from build123d import *

# Parameters (mm, degrees)
BOSS_EXTRUDE1_DEPTH     = 3.175
FILLET1_R               = 3.81
SKETCH2_R               = 2.032
CUT_EXTRUDE1_DEPTH      = 211.342252353
FILLET2_R               = 6.35
FILLET3_R               = 2.54
FILLET4_R               = 3.81
FILLET5_R               = 3.81
CUT_EXTRUDE2_DEPTH      = 211.342252353
CUT_EXTRUDE2_DEPTH_BACK = 211.342252353
FILLET6_R               = 5.08


with BuildPart() as part:
    # Sketch1 → Boss-Extrude1 (new body)
    with BuildSketch(Plane(origin=(0, 0, 0), x_dir=(1, 0, 0), z_dir=(0, 1, 0))):
        Polygon((50.8, 0), (0, 0), (0, -101.6), (50.8, -101.6), (50.8, -88.9), (63.5, -88.9), (63.5, -101.6), (120.65, -101.6), (120.65, -88.9), (133.35, -88.9), (133.35, -101.6), (184.15, -101.6), (184.15, 0), (133.35, 0), (133.35, -29.21), (120.65, -29.21), (120.65, -19.05), (63.5, -19.05), (63.5, -29.21), (50.8, -29.21), align=None)
    extrude(amount=BOSS_EXTRUDE1_DEPTH)

    # Fillet1
    fillet1_edges = [part.edges().sort_by_distance(p)[0] for p in [
        (0, 1.5875, 101.6),
        (0, 1.5875, 0),
        (184.15, 1.5875, 0),
        (184.15, 1.5875, 101.6),
    ]]
    fillet(fillet1_edges, radius=FILLET1_R)

    # Sketch2 → Cut-Extrude1 (cut, through all)
    with BuildSketch(Plane(origin=(0, 3.175, 0), x_dir=(1, 0, 0), z_dir=(0, 1, 0))):
        with Locations(Location((5.437401114, -89.146320086, 0), (0, 0, 270))):
            Circle(SKETCH2_R)
        with Locations(Location((178.712598886, -89.146320086, 0), (0, 0, 90))):
            Circle(SKETCH2_R)
        with Locations(Location((22.338907609, -48.03498858, 0), (0, 0, 270))):
            Circle(SKETCH2_R)
        with Locations(Location((15.16630044, -8.195189781, 0), (0, 0, 270))):
            Circle(SKETCH2_R)
        with Locations(Location((32.94630044, -13.97, 0), (0, 0, 270))):
            Circle(SKETCH2_R)
        with Locations(Location((32.94630044, -24.13, 0), (0, 0, 270))):
            Circle(SKETCH2_R)
        with Locations(Location((161.811092391, -48.03498858, 0), (0, 0, 90))):
            Circle(SKETCH2_R)
        with Locations(Location((151.20369956, -24.13, 0), (0, 0, 90))):
            Circle(SKETCH2_R)
        with Locations(Location((151.20369956, -13.97, 0), (0, 0, 90))):
            Circle(SKETCH2_R)
        with Locations(Location((168.98369956, -8.195189781, 0), (0, 0, 90))):
            Circle(SKETCH2_R)
    extrude(amount=-CUT_EXTRUDE1_DEPTH, mode=Mode.SUBTRACT)

    # Fillet2
    fillet2_edges = [part.edges().sort_by_distance(p)[0] for p in [
        (50.8, 1.5875, 0),
        (133.35, 1.5875, 0),
    ]]
    fillet(fillet2_edges, radius=FILLET2_R)

    # Fillet3
    fillet3_edges = [part.edges().sort_by_distance(p)[0] for p in [
        (63.5, 1.5875, 88.9),
        (50.8, 1.5875, 88.9),
        (50.8, 1.5875, 29.21),
        (63.5, 1.5875, 29.21),
        (120.65, 1.5875, 29.21),
        (133.35, 1.5875, 29.21),
        (133.35, 1.5875, 88.9),
        (120.65, 1.5875, 88.9),
    ]]
    fillet(fillet3_edges, radius=FILLET3_R)

    # Fillet4
    fillet4_edges = [part.edges().sort_by_distance(p)[0] for p in [
        (63.5, 1.5875, 19.05),
        (120.65, 1.5875, 19.05),
    ]]
    fillet(fillet4_edges, radius=FILLET4_R)

    # Fillet5
    fillet5_edges = [part.edges().sort_by_distance(p)[0] for p in [
        (63.5, 1.5875, 101.6),
        (50.8, 1.5875, 101.6),
        (133.35, 1.5875, 101.6),
        (120.65, 1.5875, 101.6),
    ]]
    fillet(fillet5_edges, radius=FILLET5_R)

    # Sketch9 → Cut-Extrude2 (cut, two sides: drawn at the far end of the back side and taken through both)
    with BuildSketch(Plane.XZ.offset(-CUT_EXTRUDE2_DEPTH_BACK)):
        with BuildLine():
            Line((147.32, 16.51), (133.35, 16.51))
            Line((133.35, 16.51), (133.35, 6.35))
            ThreePointArc((133.35, 6.35), (135.209871939, 1.859871939), (139.7, 0))
            Line((139.7, 0), (147.32, 0))
            Line((147.32, 0), (147.32, 16.51))
        make_face()
    extrude(amount=CUT_EXTRUDE2_DEPTH + CUT_EXTRUDE2_DEPTH_BACK, mode=Mode.SUBTRACT)

    # Fillet6
    fillet6_edges = [part.edges().sort_by_distance(p)[0] for p in [
        (147.32, 1.5875, 16.51),
        (147.32, 1.5875, 0),
        (133.35, 1.5875, 16.51),
    ]]
    fillet(fillet6_edges, radius=FILLET6_R)


solid = part.part
Geometry check sheet. Reference: the model listing, model coordinates, mm. A direction names the side the tool comes from. Coordinates: 2 decimals unless noted, no trailing zeros. Loops run counter-clockwise (first coordinate to the right, second up) from the corner with the lowest first, then second, coordinate; pieces in that order, holes last. Notation, with made-up numbers: (85.25, 40) - (137.25, 40) arc R20 cw to (137.25, 67) - close; hole circle Ø9 at (21, -35). An arc over 180 degrees is marked (long way). Use one line per item in the form item = value. Start each with the question number.
Item 1: Section check B-B, the plane y = 0.95. Give the number of separate pieces and of enclosed holes in the cut face, and give its area (3 significant figures).
Item 2: Gauge pin test, flat ends, axial feed: pin 1 (1.6 mm diameter, centred on x = 56, y = 2, fed in from -Z); pin 2 (1.6 mm diameter, centred on x = 140.5, y = 2, fed in from -Z); pin 3 (5.5 mm diameter, centred on x = 32.95, z = 24.13, fed in from -Y). Record the tip position at first contact, or that the pin passes through.
Item 3: Mould release check, pull along Z, two halves, no side actions. Record for faces 4 (the face through (91, 0, 50)), 5 (the face through (159.796, 1.61, 48.3)), 6 (the face through (13.36, 1.61, 9.13)), 7 (the face through (1.086, 1.61, 100.454)): +Z half, -Z half, draft (parallel to the pull), parting line (faces both ways), or undercut.
Item 4: Section check A-A, the plane z = 13.97. Enter the section's corners in (x, y) (3 decimals).
Item 5: Thickness scan on probe 1 along X at (y, z) = (1.3, 9.5); probe 2 along X at (y, z) = (1.7, 22.5); probe 3 along X at (y, z) = (1.45, 7.5). Record the ranges inside material, lowest first.
Item 6: Section check C-C, the plane x = 85.5. Enter the section's corners in (y, z) (3 decimals), and give its area (3 significant figures).
Item 7: Tool access check on faces 1 (the face through (134.799, 1.565, 18.038)), 2 (the face through (183.064, 1.61, 1.146)), 3 (the face through (120.65, 2, 95)). Record the directions out of +Z, -Z, +X, -X, +Y, -Y that give a thin tool (end or side, any length) a straight path to the whole face; none if there is none.
Computed:
q1.separate_pieces = 1
q1.enclosed_holes = 10
q1.area = 16,200 mm2
q2.pin_1 = 29.21
q2.pin_2 = 16.51
q2.pin_3 = 0
q3.face_4 = draft
q3.face_5 = undercut
q3.face_6 = undercut
q3.face_7 = +Z half
q4.outline = (0, 0) - (30.914, 0) - (30.914, 3.175) - (0, 3.175) - close; (34.978, 0) - (50.8, 0) - (50.8, 3.175) - (34.978, 3.175) - close; (146.639, 0) - (149.172, 0) - (149.172, 3.175) - (146.639, 3.175) - close; (153.236, 0) - (184.15, 0) - (184.15, 3.175) - (153.236, 3.175) - close
q5.probe_1 = 0 to 13.61, 16.72 to 50.8, 147.32 to 167.43, 170.54 to 184.15
q5.probe_2 = 0 to 31.73, 34.16 to 50.8, 63.52 to 120.63, 133.35 to 149.99, 152.42 to 184.15
q5.probe_3 = 0 to 13.26, 17.08 to 50.8, 147.32 to 167.07, 170.89 to 184.15
q6.outline = (0, 19.05) - (3.175, 19.05) - (3.175, 101.6) - (0, 101.6) - close
q6.area = 262 mm2
q7.face_1 = -Z, +Y, -Y
q7.face_2 = -Z, +X, +Y, -Y
q7.face_3 = +Z, +Y, -Y
